Drawing for the job (mm, zero at the part's lowest x, y, z). Round coordinates to 2 decimals unless told otherwise and drop trailing zeros. Loops run counter-clockwise (first coordinate to the right, second up) from the corner with the lowest first, then second, coordinate; pieces in that order, holes last. Notation, with made-up numbers: (61, 31.5) -> (94, 31.5) arc R10 ccw to (94, 37.5) -> close; hole circle Ø10 at (13, 49.25). An arc over 180 degrees is marked (long way). Put each result on its own line as item: value. Start each with the question number.
Item 1: Cut at C-C, the plane y = 2.6. Count the separate pieces of the cut face and the enclosed holes in it, plus the area to 3 significant figures.
Item 2: Cut at B-B, the plane x = 15. List the corners of the cut face in (y, z) (3 decimals).
Item 3: Drill centre lines: probe 1 along X at (y, z) = (0.9, 54); probe 2 along X at (y, z) = (1.4, 55.5); probe 3 along X at (y, z) = (2.9, 57). Where is each one in solid material? Low to high. Write a range as [from, to].
Item 4: Flat gauge pin, fed straight in: pin 1 Ø2.5 at (x, z) = (15, 15) entering from +Y. Where does the tip first touch, or does it go through?
Item 5: Cut at D-D, the plane x = 4.5. List the corners of the cut face in (y, z) (3 decimals).
Item 6: Cut at A-A, the plane z = 25. List the corners of the cut face in (x, y) (3 decimals).
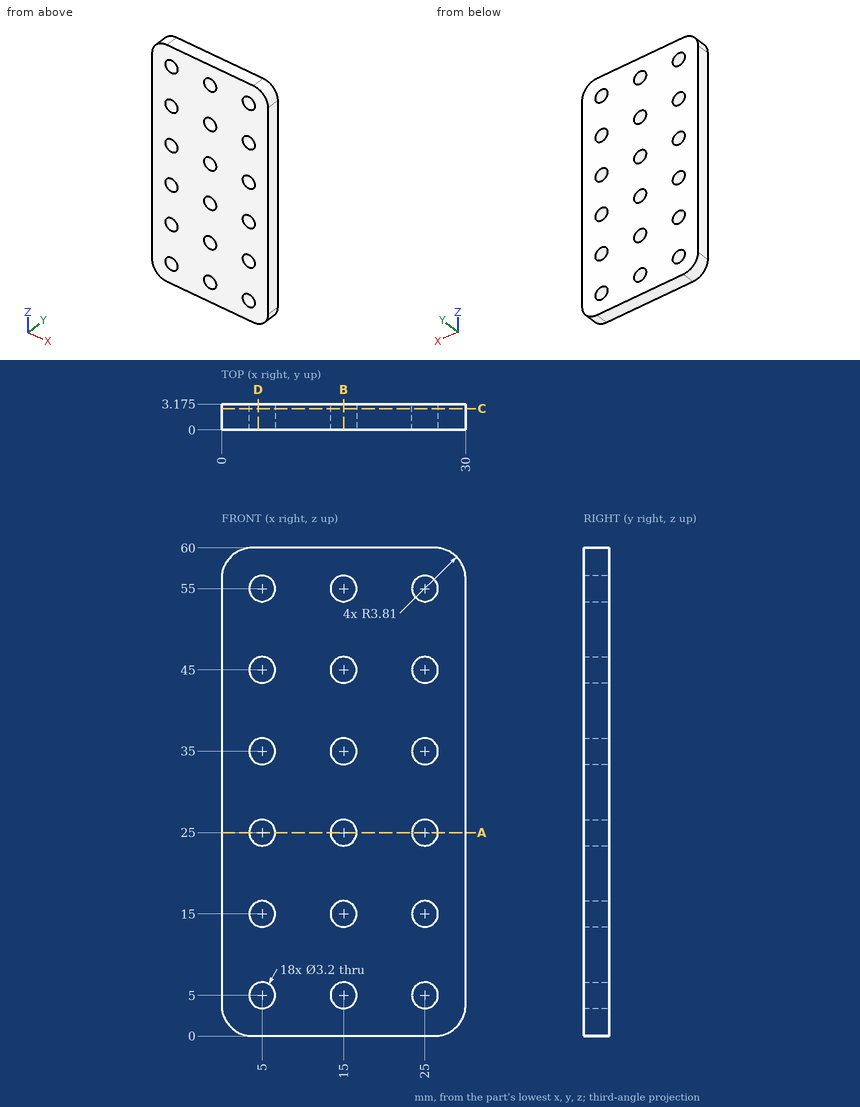
Reply:
1. separate pieces: 1
1. enclosed holes: 18
1. area: 1,640 mm^2
2. outline: (0, 0) -> (3.175, 0) -> (3.175, 3.4) -> (0, 3.4) -> close; (0, 6.6) -> (3.175, 6.6) -> (3.175, 13.4) -> (0, 13.4) -> close; (0, 16.6) -> (3.175, 16.6) -> (3.175, 23.4) -> (0, 23.4) -> close; (0, 26.6) -> (3.175, 26.6) -> (3.175, 33.4) -> (0, 33.4) -> close; (0, 36.6) -> (3.175, 36.6) -> (3.175, 43.4) -> (0, 43.4) -> close; (0, 46.6) -> (3.175, 46.6) -> (3.175, 53.4) -> (0, 53.4) -> close; (0, 56.6) -> (3.175, 56.6) -> (3.175, 60) -> (0, 60) -> close
3. probe 1: x = [0, 3.75], [6.25, 13.75], [16.25, 23.75], [26.25, 30]
3. probe 2: x = [0, 3.48], [6.52, 13.48], [16.52, 23.48], [26.52, 30]
3. probe 3: x = [0.09, 29.91]
4. pin 1: passes through
5. outline: (0, 0) -> (3.175, 0) -> (3.175, 3.48) -> (0, 3.48) -> close; (0, 6.52) -> (3.175, 6.52) -> (3.175, 13.48) -> (0, 13.48) -> close; (0, 16.52) -> (3.175, 16.52) -> (3.175, 23.48) -> (0, 23.48) -> close; (0, 26.52) -> (3.175, 26.52) -> (3.175, 33.48) -> (0, 33.48) -> close; (0, 36.52) -> (3.175, 36.52) -> (3.175, 43.48) -> (0, 43.48) -> close; (0, 46.52) -> (3.175, 46.52) -> (3.175, 53.48) -> (0, 53.48) -> close; (0, 56.52) -> (3.175, 56.52) -> (3.175, 60) -> (0, 60) -> close
6. outline: (0, 0) -> (3.4, 0) -> (3.4, 3.175) -> (0, 3.175) -> close; (6.6, 0) -> (13.4, 0) -> (13.4, 3.175) -> (6.6, 3.175) -> close; (16.6, 0) -> (23.4, 0) -> (23.4, 3.175) -> (16.6, 3.175) -> close; (26.6, 0) -> (30, 0) -> (30, 3.175) -> (26.6, 3.175) -> close
